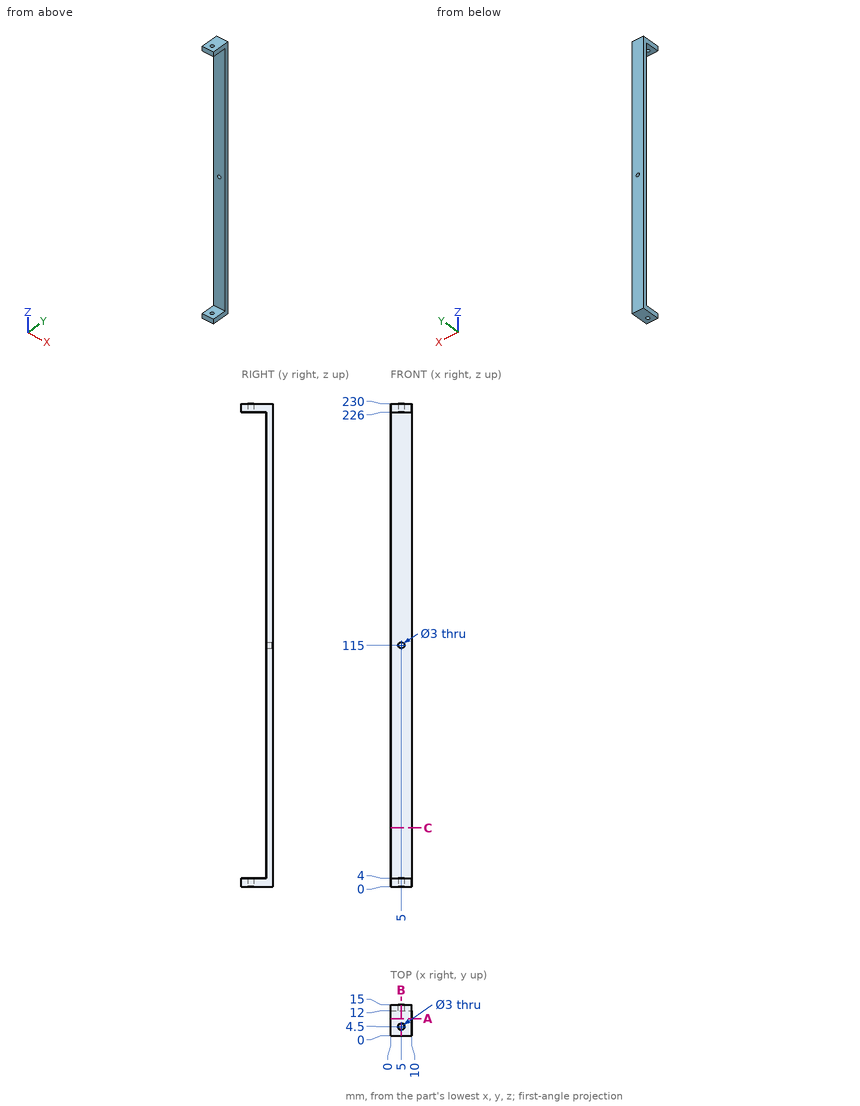
Can you work these out from the drawing? Everything is in mm from the part's minimum corner. Coordinates: 2 decimals unless noted, no trailing zeros. Loops run counter-clockwise (first coordinate to the right, second up) from the corner with the lowest first, then second, coordinate; pieces in that order, holes last. Notation, with made-up numbers: (81, -25.5) - (110, -25.5) arc R25 ccw to (110, 10.5) - close; hole circle Ø7 at (62, 23). An arc over 180 degrees is marked (long way). Put each result on its own line as item: value. Start each with the question number.
Item 1: Suppose I cut it at C-C (z = 28). Please give me the cut outline in (x, y), and give its area (3 significant figures).
Item 2: If I drill on line 1 along Z through (x, y) = (2.75, 3.5); line 2 along Y through (x, z) = (5, 0.95); line 3 along X through (y, z) = (4.5, 227.25), over which ranges is the centre line in solid material (lowest first)?
Item 3: Suppose I cut it at B-B (x = 5). Please give me the cut outline in (y, z), and give its area (3 significant figures).
Item 4: Suppose I cut it at A-A (y = 8.25). Please give me the cut outline in (x, z).
Item 5: For pin 1 (1.5 mm diameter, centred on x = 6.5, z = 154, fed in from -Y), with a flat end and sliding along its axis, tell me the tip position at first contact or that it passes through.
Here are the results:
1. outline: (0, 12) - (10, 12) - (10, 15) - (0, 15) - close
1. area: 30.0 mm²
2. line 1: 0 to 4, 226 to 230
2. line 2: 0 to 3, 6 to 15
2. line 3: 0 to 3.5, 6.5 to 10
3. outline: (0, 0) - (3, 0) - (3, 4) - (0, 4) - close; (0, 226) - (3, 226) - (3, 230) - (0, 230) - close; (6, 0) - (15, 0) - (15, 113.5) - (12, 113.5) - (12, 4) - (6, 4) - close; (6, 226) - (12, 226) - (12, 116.5) - (15, 116.5) - (15, 230) - (6, 230) - close
3. area: 753 mm²
4. outline: (0, 0) - (10, 0) - (10, 4) - (0, 4) - close; (0, 226) - (10, 226) - (10, 230) - (0, 230) - close
5. pin 1: y = 12
